from build123d import *

# Parameters (mm, degrees)
BASE_FLANGE1_DEPTH = 60
SKETCH6_R          = 11
SKETCH6_R_2        = 1.5
CUT_EXTRUDE1_DEPTH = 10
CUT_EXTRUDE2_DEPTH = 3
FILLET1_R          = 7


# Read off the part's stored shape, not the designer's step: Base-Flange1
with BuildPart() as part:
    # Base-Flange1 outline → Base-Flange1 (new body)
    with BuildSketch(Plane(origin=(0, 0, 0), x_dir=(0, 0, -1), z_dir=(1, 0, 0))):
        with BuildLine():
            Line((5, -3), (70, -3))
            Line((70, -3), (70, 0))
            Line((70, 0), (5, 0))
            ThreePointArc((5, 0), (1.464466094, 1.464466094), (0, 5))
            Line((0, 5), (0, 50))
            Line((0, 50), (-3, 50))
            Line((-3, 50), (-3, 5))
            ThreePointArc((-3, 5), (-0.656854249, -0.656854249), (5, -3))
        make_face()
    extrude(amount=BASE_FLANGE1_DEPTH)

    # Sketch6 → Cut-Extrude1 (cut)
    with BuildSketch(Plane.XY.offset(3)):
        with Locations((30, 27)):
            Circle(SKETCH6_R)
        with Locations((45.5, 42.5)):
            Circle(SKETCH6_R_2)
        with Locations(Location((14.5, 42.5, 0), (0, 0, 180))):
            Circle(SKETCH6_R_2)
        with Locations((14.5, 11.5)):
            Circle(SKETCH6_R_2)
        with Locations(Location((45.5, 11.5, 0), (0, 0, 180))):
            Circle(SKETCH6_R_2)
    extrude(amount=-CUT_EXTRUDE1_DEPTH, mode=Mode.SUBTRACT)

    # Sketch7 → Cut-Extrude2 (cut)
    with BuildSketch(Plane.XZ.offset(3)):
        with BuildLine():
            Line((6, -62.5), (6, -12.5))
            ThreePointArc((6, -12.5), (7.5, -11), (9, -12.5))
            Line((9, -12.5), (9, -62.5))
            ThreePointArc((9, -62.5), (7.5, -64), (6, -62.5))
        make_face()
        with BuildLine():
            Line((54, -62.5), (54, -12.5))
            ThreePointArc((54, -12.5), (52.5, -11), (51, -12.5))
            Line((51, -12.5), (51, -62.5))
            ThreePointArc((51, -62.5), (52.5, -64), (54, -62.5))
        make_face()
    extrude(amount=-CUT_EXTRUDE2_DEPTH, mode=Mode.SUBTRACT)

    # Fillet1
    fillet1_edges = [part.edges().sort_by_distance(p)[0] for p in [
        (60, 50, 1.5),
        (60, -1.5, -70),
        (0, 50, 1.5),
        (0, -1.5, -70),
    ]]
    fillet(fillet1_edges, radius=FILLET1_R)


solid = part.part
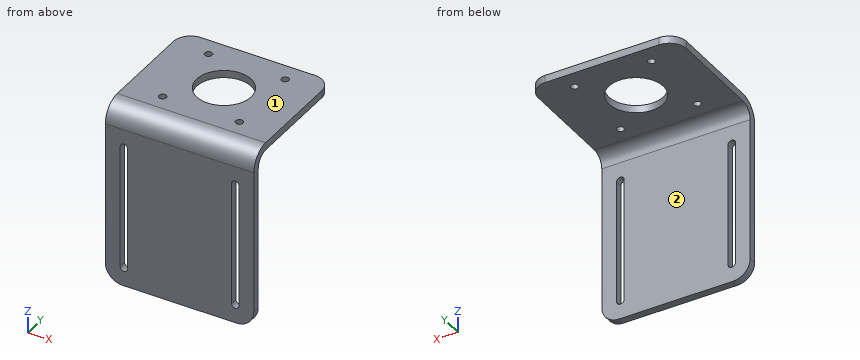
Work out the finished part from the listing and answer in its coordinate system (mm). Face numbers are marked on the shaded views. A direction names the side the tool comes from. Round coordinates to 2 decimals unless told otherwise and drop trailing zeros. Order: outer loops, then holes, each group sorted by start corner. A loop starts at its lowest first (then second) coordinate and runs counter-clockwise, first axis right, second up. Notation, with made-up numbers: M 46.25,71.25 L 87.25,71.25 A34 cw 87.25,104.25 Z; hole C 87.25,-7 d2. An arc over 180 degrees is marked long. One line per item, written item: value.
Q1. Straight lines are drawn through the part: line 1 (Y direction, x = 45, z = 2); line 2 (Y direction, x = 45.5, z = 1.7); line 3 (Z direction, x = 11.5, y = 30). For each, find the intervals that lie inside material, in ascending order.
Derived:
line 1: 1.13 to 10.09, 12.91 to 41.09, 43.91 to 50
line 2: 0.63 to 10, 13 to 41, 44 to 50
line 3: 0 to 3
Q2. Find section C-C on x = 46. Write down the section's boundary in (y, z).
Derived:
outline: M -3,-70 L 0,-70 L 0,-5 A5 cw 5,0 L 10.09,0 L 10.09,3 L 5,3 A8 ccw -3,-5 Z; M 12.91,0 L 41.09,0 L 41.09,3 L 12.91,3 Z; M 43.91,0 L 50,0 L 50,3 L 43.91,3 Z
Q3. Flat-ended cylindrical pins translate along their axes: pin 1 (1.8 mm diameter, centred on x = 45.5, y = 42.5, fed in from +Z); pin 2 (8 mm diameter, centred on x = 44.5, z = -6.5, fed in from +Y); pin 3 (1.5 mm diameter, centred on x = 15, y = 12.5, fed in from -Z); pin 4 (18 mm diameter, centred on x = 21.5, z = -31, fed in from +Y). Find the tip coordinate at first contact, or state that the pin passes through.
Derived:
pin 1: through
pin 2: y = 0.67
pin 3: z = 0
pin 4: y = 0
Q4. For the marked faces 1 and 2, determine the directions among +Z, -Z, +X, -X, +Y, -Y from which every point of the face is accessible in a straight line to the end or side of a thin tool.
Derived:
face 1: +Z, +X, -X, +Y, -Y
face 2: -Z, +X, -X, +Y
Q5. Find section A-A on z = -47.5. Write down the section's boundary in (x, y), then the cut area to 3 significant figures.
Derived:
outline: M 0,-3 L 6,-3 L 6,0 L 0,0 Z; M 9,-3 L 51,-3 L 51,0 L 9,0 Z; M 54,-3 L 60,-3 L 60,0 L 54,0 Z
area: 162 mm²
Q6. Find section B-B on x = 30. Write down the section's boundary in (y, z).
Derived:
outline: M -3,-70 L 0,-70 L 0,-5 A5 cw 5,0 L 16,0 L 16,3 L 5,3 A8 ccw -3,-5 Z; M 38,0 L 50,0 L 50,3 L 38,3 Z
Q7. Find section D-D on y = 18. Write down the section's boundary in (x, z), then the cut area to 3 significant figures.
Derived:
outline: M 0,0 L 23.68,0 L 23.68,3 L 0,3 Z; M 36.32,0 L 60,0 L 60,3 L 36.32,3 Z
area: 142 mm²
